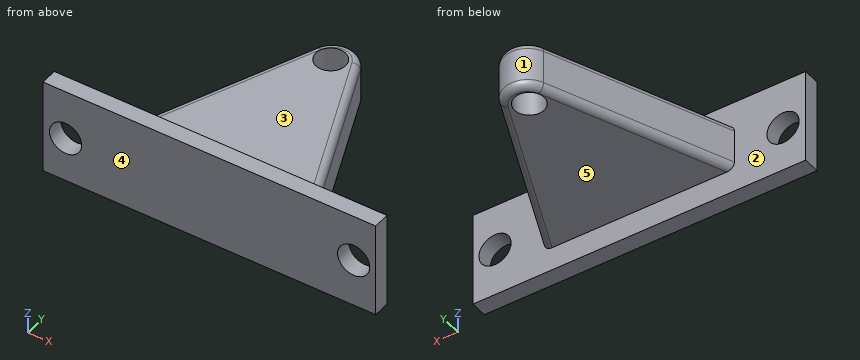
Autodesk Fusion 360 part; units mm, degrees
sketch "Sketch1" plane through (0, 0, 0) normal (0, 0, 1) x (1, 0, 0)
  line L0 (-40, 0) -> (-0.4355, 95.3806)
  line L1 (-0.4355, 95.3806) -> (40, 0)
  line L2 (40, 0) -> (-40, 0)
extrude "Extrude1" add sketch "Sketch1" along normal blind 20
hole "Hole1" at (-0.9754, 69.5316, 20) direction (0, 0, -1) diameter 12.5 depth 40 tip angle 118
fillet "Fillet1" radius 10 1 edges at (-0.4355, 95.3806, 10)
sketch "Sketch2" plane through (0, 0, 0) normal (0, 1, 0) x (1, 0, 0)
  line L0 (-70, -30) -> (70, -30)
  line L1 (70, -30) -> (70, 10)
  line L2 (70, 10) -> (-70, 10)
  line L3 (-70, 10) -> (-70, -30)
extrude "Extrude2" add sketch "Sketch2" against normal blind 7
hole "Hole2" at (60.7368, 0, 10.2504) direction (0, -1, 0) diameter 13.53 depth 20 tip angle 118
hole "Hole3" at (-60.4864, 0, 8.9986) direction (0, -1, 0) diameter 13.53 depth 20 tip angle 118
fillet "Fillet2" radius 3 6 edges at (-24.786, 36.6774, 20) (-0.3739, 79.5232, 20) (24.4359, 36.7132, 20) (-24.786, 36.6774, 0) (-0.3739, 79.5232, 0) (24.4359, 36.7132, 0)
For this review, take the finished solid that the model builds, in its own axes (mm). Face numbers are marked on the shaded views. A direction names the side the tool comes from. Coordinates: 2 decimals unless noted, no trailing zeros. Write each loop counter-clockwise with the first axis right and the second up, starting at its lowest first coordinate (ties: lowest second). Pieces come first, ordered by that corner, then holes.
(1) Add section B-B on x = -44.5. Give the boundary of the cut face in (y, z), then the cut area to 3 significant figures.
(2) Tool access review of the marked faces 1 and 2: name each direction out of +Z, -Z, +X, -X, +Y, -Y from which nothing blocks a thin tool from reaching the whole face with its end or side.
(3) Wall thickness on probe 1 along Y at (x, z) = (40.5, 23); probe 2 along Z at (x, y) = (-1.5, 26.5); probe 3 along X at (y, z) = (64.5, 1.5): over which ranges is each line inside the solid? List them lowest first.
(4) For pin 1 Ø12 at (x, y) = (22, 31) entering from -Z; pin 2 Ø6 at (y, z) = (64.5, 16.5) entering from -X; pin 3 Ø10 at (y, z) = (35.5, -4.5) entering from +X; pin 4 Ø20 at (x, z) = (4, 4.5) entering from +Y, all flat-tipped, find the tip position at first contact; note any pin that passes through.
(5) Add section C-C on z = -4. Give the boundary of the cut face in (x, y), then the cut area to 3 significant figures.
(6) The part is to be moulded in two halves that separate along Z. For the marked faces 3, 4 and 5, say which applies: +Z half, -Z half, draft (parallel to the pull), parting line (faces both ways), or undercut.
(7) Add section A-A on z = 10.5. Give the boundary of the cut face in (x, y).
Answer sheet:
1. outline: (-7, -10) - (0, -10) - (0, 30) - (-7, 30) - close
1. area: 280 mm2
2. face 1: +Z, -Z, +Y
2. face 2: +Y
3. probe 1: y = -7 to 0
3. probe 2: z = 0 to 20
3. probe 3: x = -12.81 to -4.68, 2.73 to 12.22
4. pin 1: stops at z = 0
4. pin 2: stops at x = -14.49
4. pin 3: stops at x = 23.74
4. pin 4: stops at y = 79.52
5. outline: (-70, -7) - (70, -7) - (70, 0) - (-70, 0) - close
5. area: 980 mm2
6. face 3: +Z half
6. face 4: draft
6. face 5: -Z half
7. outline: (-70, -7) - (-67.08, -7) - (-67.08, 0) - (-70, 0) - close; (-53.89, -7) - (53.98, -7) - (53.98, 0) - (40, 0) - (8.87, 73.43) arc R10 ccw to (-9.57, 73.35) - (-40, 0) - (-53.89, 0) - close; (67.5, -7) - (70, -7) - (70, 0) - (67.5, 0) - close; hole circle Ø12.5 at (-0.98, 69.53)
